from build123d import *

# Parameters (mm, degrees)
SKETCH1_W           = 80
SKETCH1_H           = 8
BOSS_EXTRUDE1_DEPTH = 30
FILLET1_R           = 7
FILLET2_R           = 7
BOSS_EXTRUDE3_DEPTH = 30
SKETCH4_W           = 18
SKETCH4_H           = 26
CUT_EXTRUDE1_DEPTH  = 26
SKETCH5_R           = 12
BOSS_EXTRUDE4_DEPTH = 32
BOSS_EXTRUDE5_START = 2
SKETCH6_R           = 12
BOSS_EXTRUDE5_DEPTH = 2
CUT_EXTRUDE2_REACH  = 76.983
SKETCH7_R           = 6
CUT_EXTRUDE3_REACH  = 69.701
SKETCH8_R           = 4


with BuildPart() as part:
    # Sketch1 → Boss-Extrude1 (new body)
    with BuildSketch(Plane(origin=(0, 0, 0), x_dir=(0, 0, -1), z_dir=(1, 0, 0))):
        with Locations((-5.989847716, 6.487309645)):
            Rectangle(SKETCH1_W, SKETCH1_H)
    extrude(amount=-BOSS_EXTRUDE1_DEPTH)

    # Fillet1
    fillet1_edges = [part.edges().sort_by_distance(p)[0] for p in [
        (0, 6.487309645, 45.989847716),
    ]]
    fillet(fillet1_edges, radius=FILLET1_R)

    # Fillet2
    fillet2_edges = [part.edges().sort_by_distance(p)[0] for p in [
        (-30, 6.487309645, 45.989847716),
    ]]
    fillet(fillet2_edges, radius=FILLET2_R)

    # Sketch2 → Boss-Extrude3 (add)
    with BuildSketch(Plane(origin=(0, 0, 0), x_dir=(0, 0, -1), z_dir=(1, 0, 0))):
        with BuildLine():
            Line((-17.989847716, 10.487309645), (-17.989847716, 36.487309645))
            ThreePointArc((-17.989847716, 36.487309645), (-11.995980002, 46.878521813), (0, 46.892814939))
            Line((0, 46.892814939), (34.010152284, 10.487309645))
            Line((34.010152284, 10.487309645), (-17.989847716, 10.487309645))
        make_face()
    extrude(amount=-BOSS_EXTRUDE3_DEPTH)

    # Sketch4 → Cut-Extrude1 (cut)
    with BuildSketch(Plane.XY.offset(17.989847716)):
        with Locations((-15, 23.487309645)):
            Rectangle(SKETCH4_W, SKETCH4_H)
    extrude(amount=-CUT_EXTRUDE1_DEPTH, mode=Mode.SUBTRACT)

    # Sketch5 → Boss-Extrude4 (add)
    with BuildSketch(Plane(origin=(0, 0, 0), x_dir=(0, 0, -1), z_dir=(1, 0, 0))):
        with Locations((-5.985600429, 36.487309645)):
            Circle(SKETCH5_R)
    extrude(amount=-BOSS_EXTRUDE4_DEPTH)

    # Sketch6 → Boss-Extrude5 (add)
    with BuildSketch(Plane(origin=(0, 0, 0), x_dir=(0, 0, -1), z_dir=(1, 0, 0)).offset(BOSS_EXTRUDE5_START)):
        with Locations((-5.985600429, 36.487309645)):
            Circle(SKETCH6_R)
    extrude(amount=-BOSS_EXTRUDE5_DEPTH)

    # Sketch7 → Cut-Extrude2 (cut, up to next)
    with BuildSketch(Plane(origin=(2, 0, 0), x_dir=(0, 0, -1), z_dir=(1, 0, 0)), mode=Mode.PRIVATE) as cut_extrude2_sk1:
        with Locations((-5.985600429, 36.487309645)):
            Circle(SKETCH7_R)
    cut_extrude2_tool1 = extrude(cut_extrude2_sk1.sketch, amount=-CUT_EXTRUDE2_REACH, mode=Mode.PRIVATE) & part.part
    add(cut_extrude2_tool1.solids().sort_by_distance((2, 36.48731, 5.9856))[0], mode=Mode.SUBTRACT)

    # Sketch8 → Cut-Extrude3 (cut, up to next)
    with BuildSketch(Plane(origin=(0, 10.487309645, 0), x_dir=(1, 0, 0), z_dir=(0, 1, 0)), mode=Mode.PRIVATE) as cut_extrude3_sk1:
        with Locations(Location((-15, -38.989847716, 0), (0, 0, 270))):
            Circle(SKETCH8_R)
    cut_extrude3_tool1 = extrude(cut_extrude3_sk1.sketch, amount=-CUT_EXTRUDE3_REACH, mode=Mode.PRIVATE) & part.part
    add(cut_extrude3_tool1.solids().sort_by_distance((-15, 10.48731, 38.989848))[0], mode=Mode.SUBTRACT)


solid = part.part
Could you check a few things on this model? Use its own coordinates, in mm. A direction names the side the tool comes from. Give positions to 0.01 mm unless a question says otherwise; leave off trailing zeros. Order: outer loops, then holes, each group sorted by start corner. A loop starts at its lowest first (then second) coordinate and runs counter-clockwise, first axis right, second up.
1. Suppose I cut it at B-B (y = 7.5). Write out the boundary of the cut face in (x, z).
Answers below:
outline: (-30, -34.01) - (0, -34.01) - (0, 38.99) arc R7 ccw to (-7, 45.99) - (-23, 45.99) arc R7 ccw to (-30, 38.99) - close; hole circle Ø8 at (-15, 38.99)
2. Suppose I cut it at A-A (x = -15). State how many separate pieces and enclosed holes the cut face has, plus the area to 3 significant figures.
Answers below:
separate pieces: 2
enclosed holes: 1
area: 1,280 mm2
3. Suppose I cut it at D-D (z = 37). Write out the boundary of the cut face in (x, y), plus the area to 3 significant figures.
Answers below:
outline: (-30, 2.49) - (-18.47, 2.49) - (-18.47, 10.49) - (-30, 10.49) - close; (-11.53, 2.49) - (0, 2.49) - (0, 10.49) - (-11.53, 10.49) - close
area: 184 mm2
4. Thinking about a two-plate mould opening in Y: for faces 1 (the cylindrical face through (-14.87, 24.49, 6.25)), 2 (the cylindrical face through (-14.79, 46.79, 12.15)), 3 (the cylindrical face through (-27.9, 6.54, 43.99)), which applies, +Y half, -Y half, draft (parallel to the pull), parting line (faces both ways), or undercut?
Answers below:
face 1: undercut
face 2: +Y half
face 3: draft
5. I need wall thicknesses on L1, parallel to Y at x = -21, z = 0.5; L2, parallel to Z at x = -17, y = 35; L3, parallel to Y at x = -18.5, z = 7. Which ranges of each line are inside material? Lowest first, please.
Answers below:
L1: y = 2.49 to 10.49, 25.81 to 34.06, 38.92 to 47.16
L2: z = -11.11 to -8.01, -5.92 to 0.17, 11.8 to 17.89
L3: y = 2.49 to 10.49, 24.53 to 30.57, 42.4 to 48.45
6. Which directions (+Z, -Z, +X, -X, +Y, -Y) give clear straight access to the entire face, cutting with the end or side of a thin tool? Please do faces 4 (the flat face through (-27, 23, 17.99)), 5 (the flat face through (-15, 10.487, 19)), 6 (the flat face through (-15, 36.487, -7)).
Answers below:
face 4: +Z, +X, -X, +Y
face 5: +Z
face 6: none
7. For pin 1 (4 mm diameter, centred on y = 16, z = -21.5, fed in from +X); pin 2 (10 mm diameter, centred on x = -11, z = 32, fed in from +Y); pin 3 (5 mm diameter, centred on x = -4.5, y = 29, fed in from +Z); pin 4 (9.5 mm diameter, centred on y = 36.49, z = 5.99, fed in from -X), each with a flat end and sliding along its axis, tell me the tip position at first contact or that it passes through.
Answers below:
pin 1: stops at x = 0
pin 2: stops at y = 10.49
pin 3: stops at z = 17.99
pin 4: passes through
